```python
from build123d import *

# Parameters (mm, degrees)
F0_W     = 60
F0_H     = 30
F1_DEPTH = 3
F2_W     = 60
F2_H     = 8.6
F2_R     = 5
F2_R_2   = 1.5
F3_DEPTH = 7
F4_R     = 0.5


with BuildPart() as f1:
    # F0 (on Top) → F1 (new body)
    with BuildSketch(Plane.XY):
        Rectangle(F0_W, F0_H)
    extrude(amount=F1_DEPTH)

    # F2 (on face) → F3 (join)
    with BuildSketch(Plane.XY.offset(3)):
        with Locations((0, 10.7)):
            Rectangle(F2_W, F2_H)
        with Locations((-7.5, 0)):
            Circle(F2_R)
        with Locations((-7.5, 0)):
            Circle(F2_R_2, mode=Mode.SUBTRACT)
        with Locations((7.5, 0)):
            Circle(F2_R)
        with Locations((7.5, 0)):
            Circle(F2_R_2, mode=Mode.SUBTRACT)
        with BuildLine():
            Line((-18.2, 4.3), (-30, 4.3))
            Line((-30, 4.3), (-30, -15))
            Line((-30, -15), (30, -15))
            Line((30, -15), (30, 4.3))
            Line((30, 4.3), (18.2, 4.3))
            ThreePointArc((18.2, 4.3), (15.159441, 3.040559), (13.9, 0))
            ThreePointArc((13.9, 0), (12.025483, -4.525483), (7.5, -6.4))
            Line((7.5, -6.4), (-7.5, -6.4))
            ThreePointArc((-7.5, -6.4), (-12.025483, -4.525483), (-13.9, 0))
            ThreePointArc((-13.9, 0), (-15.159441, 3.040559), (-18.2, 4.3))
        make_face()
    extrude(amount=F3_DEPTH)

    # F4
    f4_edges = [f1.edges().sort_by_distance(p)[0] for p in [
        (-15.159441, 3.040559, 10),
        (-24.1, 4.3, 10),
        (-30, -5.35, 10),
        (0, -15, 10),
        (30, -5.35, 10),
        (24.1, 4.3, 10),
        (15.159441, 3.040559, 10),
        (12.025483, -4.525483, 10),
        (0, -6.4, 10),
        (-12.025483, -4.525483, 10),
        (0, 15, 10),
        (-30, 10.7, 10),
        (0, 6.4, 10),
        (30, 10.7, 10),
        (-12.5, 0, 10),
        (-9, 0, 10),
        (2.5, 0, 10),
        (6, 0, 10),
    ]]
    fillet(f4_edges, radius=F4_R)


solid = f1.part
```
Here's how the part is built. I have some questions about the finished solid (model axes, mm). A direction names the side the tool comes from. Round coordinates to 2 decimals unless told otherwise and drop trailing zeros. Write each loop counter-clockwise with the first axis right and the second up, starting at its lowest first coordinate (ties: lowest second). Pieces come first, ordered by that corner, then holes.
Q1. Which directions (+Z, -Z, +X, -X, +Y, -Y) give clear straight access to the entire face, cutting with the end or side of a thin tool? Please do faces 1 (the flat face through (0, 6.4, 6)), 2 (the cylindrical face through (15.19, 3.07, 6.2)), 3 (the flat face through (0, -15, 5)).
Q2. Will this pin go through, and if not, where does the flat tip stop? P1, Ø1.8, axis at x = -7.5, y = 0, coming from the +Z side.
Q3. If we section it at B-B on x = 0: Write out the boundary of the cut face in (y, z).
Q4. If we section it at A-A on z = 5: Write out the boundary of the cut face in (x, y), plus the area to 3 significant figures.
Q5. If we mould it in two halves opening along X, with no side actions, what happens to faces 4 (the cylindrical face through (-11.98, -4.57, 6.2)), 5 (the flat face through (-8, 0, 3)), 6 (the flat face through (30, 0, 5)), 7 (the flat face through (9.44, -0.94, 10))? For each: +X half, -X half, draft (parallel to the pull), parting line (faces both ways), or undercut.
Q6. Please list where these lines run through material, in increasing order: probe 1 along Y at (x, z) = (-7.5, 7.75); probe 2 along Y at (x, z) = (-20.5, 5.5); probe 3 along Y at (x, z) = (2, 4.5).
Answer below:
1. face 1: +Z, +X, -X
1. face 2: +Z
1. face 3: +Z, -Z, +X, -X, -Y
2. P1: stops at z = 3
3. outline: (-15, 0) - (15, 0) - (15, 9.5) arc R0.5 ccw to (14.5, 10) - (6.9, 10) arc R0.5 ccw to (6.4, 9.5) - (6.4, 3) - (-6.4, 3) - (-6.4, 9.5) arc R0.5 ccw to (-6.9, 10) - (-14.5, 10) arc R0.5 ccw to (-15, 9.5) - close
4. outline: (-30, -15) - (30, -15) - (30, 4.3) - (18.2, 4.3) arc R4.3 ccw to (13.9, 0) arc R6.4 cw to (7.5, -6.4) - (-7.5, -6.4) arc R6.4 cw to (-13.9, 0) arc R4.3 ccw to (-18.2, 4.3) - (-30, 4.3) - close; (-30, 6.4) - (30, 6.4) - (30, 15) - (-30, 15) - close; circle Ø10 at (-7.5, 0); circle Ø10 at (7.5, 0); hole circle Ø3 at (-7.5, 0); hole circle Ø3 at (7.5, 0)
4. area: 1,530 mm2
5. face 4: undercut
5. face 5: undercut
5. face 6: +X half
5. face 7: draft
6. probe 1: y = -15 to -6.4, -5 to -1.5, 1.5 to 5, 6.4 to 15
6. probe 2: y = -15 to 4.3, 6.4 to 15
6. probe 3: y = -15 to -6.4, 6.4 to 15
